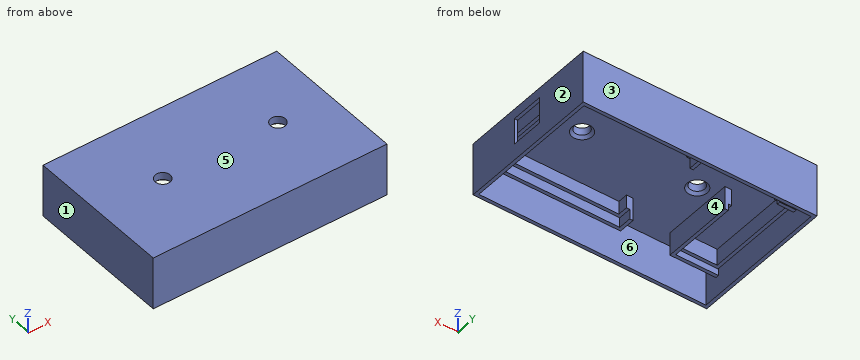
from build123d import *

# Parameters (mm, degrees)
SKETCH033_W         = 71
SKETCH033_H         = 44
PAD022_DEPTH        = 3
HOLE003_D           = 4.5
HOLE003_DEPTH       = 25
HOLE003_CSINK_D     = 6.1
HOLE003_CSINK_ANGLE = 90
PAD023_DEPTH        = 7
SKETCH036_W         = 71
SKETCH036_H         = 44
SKETCH036_W_2       = 69
SKETCH036_H_2       = 42
PAD024_DEPTH        = 13
PAD025_DEPTH        = 7
SKETCH_W            = 10
SKETCH_H            = 8
POCKET005_DEPTH     = 5
PAD026_DEPTH        = 5
PAD029_DEPTH        = 4


with BuildPart() as part:
    # Sketch033 → Pad022 (new body)
    with BuildSketch(Plane.XY):
        with Locations((35.5, 22)):
            Rectangle(SKETCH033_W, SKETCH033_H)
    extrude(amount=-PAD022_DEPTH)

    # Hole003
    with Locations(Plane(origin=(0, 0, -3), x_dir=(1, 0, 0), z_dir=(0, 0, -1))):
        with Locations((20, -22.5), (55, -22.5)):
            CounterSinkHole(HOLE003_D / 2, HOLE003_CSINK_D / 2, depth=HOLE003_DEPTH, counter_sink_angle=HOLE003_CSINK_ANGLE)

    # Sketch035 → Pad023 (join)
    with BuildSketch(Plane.XY.offset(-3)):
        Polygon((71, 39), (30, 39), (30, 34), (31, 34), (31, 38), (70, 38), (70, 6), (31, 6), (31, 10), (30, 10), (30, 5), (71, 5), align=None)
    extrude(amount=-PAD023_DEPTH)

    # Sketch036 → Pad024 (join)
    with BuildSketch(Plane.XY.offset(-3)):
        with Locations((35.5, 22)):
            Rectangle(SKETCH036_W, SKETCH036_H)
        with Locations((35.5, 22)):
            Rectangle(SKETCH036_W_2, SKETCH036_H_2, mode=Mode.SUBTRACT)
    extrude(amount=-PAD024_DEPTH)

    # Sketch038 → Pad025 (join)
    with BuildSketch(Plane.XY.offset(-3)):
        Polygon((6, 37), (6, 36), (1, 36), (1, 6), (14, 6), (14, 27), (15, 27), (15, 5), (0, 5), (0, 37), align=None)
    extrude(amount=-PAD025_DEPTH)

    # Sketch (on Face9 of Pad025) → Pocket005 (cut)
    with BuildSketch(Plane.YZ.offset(71)):
        with Locations((21.5, -7)):
            Rectangle(SKETCH_W, SKETCH_H)
    extrude(amount=-POCKET005_DEPTH, mode=Mode.SUBTRACT)

    # Sketch039 → Pad026 (join)
    with BuildSketch(Plane.XY.offset(-3)):
        Polygon((6, 36), (1.15, 36), (1.15, 6), (14, 6), (14, 27), (13, 27), (13, 7), (2.15, 7), (2.15, 35), (6, 35), align=None)
    extrude(amount=-PAD026_DEPTH)

    # Sketch042 → Pad029 (join)
    with BuildSketch(Plane.XY.offset(-3)):
        Polygon((31, 10), (31, 6), (70, 6), (70, 38), (31, 38), (31, 34), (32, 34), (32, 37), (69, 37), (69, 7), (32, 7), (32, 10), align=None)
    extrude(amount=-PAD029_DEPTH)


with BuildPart() as part_1:
    # Body011 placement: moved
    add(part.part.moved(Location((3, 3, 17))))


solid = part_1.part
Source: CAD feature listing. Evaluate the final solid. Frame: model axes, mm. Face numbers are marked on the shaded views. A direction names the side the tool comes from. Coordinates: 2 decimals unless noted, no trailing zeros. Order: outer loops, then holes, each group sorted by start corner. A loop starts at its lowest first (then second) coordinate and runs counter-clockwise, first axis right, second up. Notation, with made-up numbers: M -26,50 L 6,50 A11 ccw 6,58 Z; hole C 87.25,83 d1. An arc over 180 degrees is marked long. Write each question's results on one line, items separated by ' | '. Start each with the question number.
Item 1: Draft query along X for the marked faces 1, 2, 3 and 4. Return one class per face: pulls with the +X half, pulls with the -X half, needs draft (parallel to the pull), parting line crosses it, or undercut.
Item 2: Set-up query: the marked faces 5 and 6. Return all of +Z, -Z, +X, -X, +Y, -Y with unobstructed straight access to the full face (end or side cutting, diameter ignored); none if empty.
Item 3: Line query: probe 1 along Y at (x, z) = (40, 13.75); probe 2 along Y at (x, z) = (10.5, 8.75); probe 3 along X at (y, z) = (25.5, 15.3). Output: solid intervals per line, ascending.
Item 4: Cut plane D-D (x = 63). Return loops of the section in (y, z), and give its area (3 significant figures).
Item 5: Cut plane B-B (x = 23). Return loops of the section in (y, z), and give its area (3 significant figures).
Item 6: Cut plane A-A (y = 21.5). Return loops of the section in (x, z).
Item 7: Cut plane C-C (z = 2.5). Return loops of the section in (x, y).
Item 8: First-contact query: pin 1 Ø7 at (x, y) = (23, 25.5) entering from -Z; pin 2 Ø12.5 at (x, y) = (34.5, 31.5) entering from -Z. Flat tips, straight axial feed; report the tip coordinate or a pass-through.
Checked values:
1) face 1: pulls with the -X half | face 2: pulls with the +X half | face 3: needs draft | face 4: undercut
2) face 5: +Z, +X, -X, +Y, -Y | face 6: -Z
3) probe 1: y = 3 to 4, 8 to 10, 40 to 42, 46 to 47 | probe 2: y = 3 to 4, 8 to 9, 46 to 47 | probe 3: x = 3 to 20.75, 25.25 to 55.75, 60.25 to 74
4) outline: M 3,1 L 4,1 L 4,14 L 8,14 L 8,7 L 9,7 L 9,10 L 10,10 L 10,14 L 40,14 L 40,10 L 41,10 L 41,7 L 42,7 L 42,14 L 46,14 L 46,1 L 47,1 L 47,17 L 3,17 Z | area: 180 mm2
5) outline: M 3,1 L 4,1 L 4,14 L 22.45,14 L 23.25,14.8 L 23.25,17 L 3,17 Z; M 27.75,14.8 L 28.55,14 L 46,14 L 46,1 L 47,1 L 47,17 L 27.75,17 Z | area: 144 mm2
6) outline: M 3,1 L 4,1 L 4,14 L 4.15,14 L 4.15,9 L 5.15,9 L 5.15,14 L 16,14 L 16,9 L 17,9 L 17,7 L 18,7 L 18,14 L 72,14 L 72,10 L 73,10 L 73,14 L 74,14 L 74,17 L 3,17 Z; M 73,1 L 74,1 L 74,6 L 73,6 Z
7) outline: M 3,3 L 74,3 L 74,47 L 3,47 Z; hole M 4,4 L 73,4 L 73,46 L 4,46 Z
8) pin 1: stops at z = 14 | pin 2: stops at z = 7
